Design review of the part shown in the three views and the two pictorial views. Dimensions are in mm from the part's minimum x, y and z. A direction names the side the tool comes from. Give positions to 0.01 mm unless a question says otherwise; leave off trailing zeros. Order: outer loops, then holes, each group sorted by start corner. A loop starts at its lowest first (then second) coordinate and runs counter-clockwise, first axis right, second up.
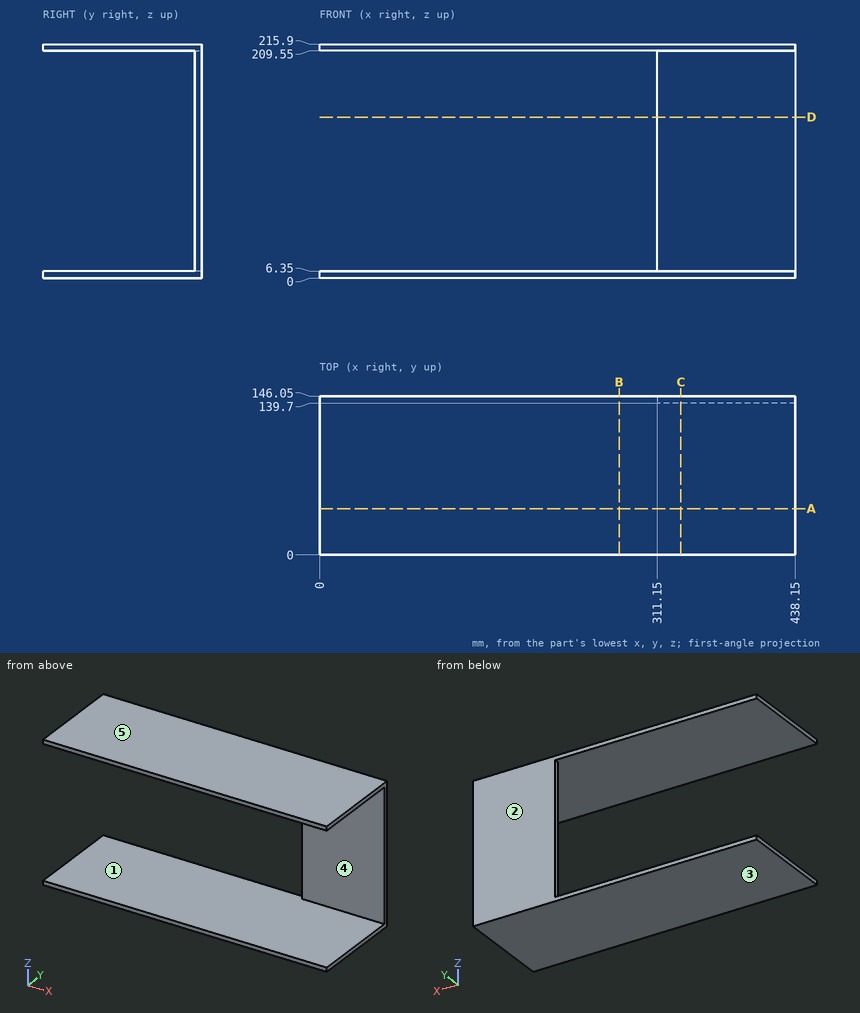
Item 1: Take a section at A-A (y = 42.5). Give the boundary of the cut face in (x, z), and give its area (3 significant figures).
Values found:
outline: (0, 0) - (438.15, 0) - (438.15, 6.35) - (0, 6.35) - close; (0, 209.55) - (438.15, 209.55) - (438.15, 215.9) - (0, 215.9) - close
area: 5,560 mm2
Item 2: Take a section at B-B (x = 276). Give the boundary of the cut face in (y, z), and give its area (3 significant figures).
Values found:
outline: (0, 0) - (146.05, 0) - (146.05, 6.35) - (0, 6.35) - close; (0, 209.55) - (146.05, 209.55) - (146.05, 215.9) - (0, 215.9) - close
area: 1,850 mm2
Item 3: Take a section at D-D (z = 148.5). Give the boundary of the cut face in (x, y).
Values found:
outline: (311.15, 139.7) - (438.15, 139.7) - (438.15, 146.05) - (311.15, 146.05) - close
Item 4: Take a section at C-C (x = 333). Give the boundary of the cut face in (y, z).
Values found:
outline: (0, 0) - (146.05, 0) - (146.05, 215.9) - (0, 215.9) - (0, 209.55) - (139.7, 209.55) - (139.7, 6.35) - (0, 6.35) - close
Item 5: Clearance check with flat-ended pins moving along their axes: pin 1 Ø1.9 at (y, z) = (141.5, 91) entering from -X; pin 2 Ø4 at (x, z) = (376, 27.5) entering from -Y. State where each tip first meets the part, or that it passes through.
Values found:
pin 1: stops at x = 311.15
pin 2: stops at y = 139.7
Item 6: Draft analysis for pull direction Z (two halves, no side actions). For the marked faces 1, 2 and 3, state which applies: released by +Z, released by -Z, zero draft, split by the parting line, or undercut.
Values found:
face 1: undercut
face 2: zero draft
face 3: released by -Z
Item 7: For line 1 (Z direction, x = 100, y = 104); line 2 (Y direction, x = 360.5, z = 97.5), list the stretches that pass through material, from the lowest coordinate up.
Values found:
line 1: z = 0 to 6.35, 209.55 to 215.9
line 2: y = 139.7 to 146.05
Item 8: For the marked faces 4 and 5, list the 3-axis set-ups (+Z, -Z, +X, -X, +Y, -Y) from which the entire face can be reached by the end or side of a thin tool; tool diameter is ignored.
Values found:
face 4: +X, -X, -Y
face 5: +Z, +X, -X, +Y, -Y
